Read the model definition and answer for the solid it produces. Units are mm, in the model's axes. Face numbers are marked on the shaded views. A direction names the side the tool comes from. Coordinates: 2 decimals unless noted, no trailing zeros. Write each loop counter-clockwise with the first axis right and the second up, starting at its lowest first coordinate (ties: lowest second). Pieces come first, ordered by that corner, then holes. Notation, with made-up numbers: (23, -7.5) -> (39, -7.5) arc R27 ccw to (39, 30.5) -> close; hole circle Ø8 at (54.25, -21). An arc over 180 degrees is marked (long way). Answer in a Markdown table with one row per item. Add a question column.
Item 1: For a pull along Y with two mould halves and no side action, classify the marked faces 5, 6, 7 and 8 as +Y half, -Y half, draft (parallel to the pull), parting line (faces both ways), or undercut.
Item 2: Which of the six approach directions +Z, -Z, +X, -X, +Y, -Y give full straight-line access (tool end or side, diameter ignored) to the marked faces 1, 2, 3 and 4?
Item 3: Given pin 1 Ø1.5 at (y, z) = (-1.5, 4) entering from -X; pin 2 Ø3.5 at (y, z) = (15, 4) entering from -X; pin 3 Ø3 at (x, z) = (5.5, 4) entering from -Y, each flat-ended and moving along its own axis, determine where each tip first touches the part or whether it passes through.
Item 4: Section A-A on x = 4.8 is taken. Write down the section's boundary in (y, z).
Item 5: Section D-D on z = 3.5 is taken. Count the separate pieces of the cut face and the enclosed holes in it, then the cut area to 3 significant figures.
Item 6: Section C-C on y = 0 is taken. Write down the section's boundary in (x, z).
Item 7: Section B-B on y = 18.5 is taken. Write down the section's boundary in (x, z).
Item 8: Straight lines are drawn through the part: line 1 (Z direction, x = 4.8, y = 13.25); line 2 (Y direction, x = -0.25, z = 2.25); line 3 (Y direction, x = 8, z = 0.75). For each, find the intervals that lie inside material, in ascending order. Write a range as from..to.
```python
from build123d import *

# Parameters (mm, degrees)
BOSS_EXTRUDE1_DEPTH = 8
SKETCH2_R           = 1.65
CUT_EXTRUDE1_DEPTH  = 18
CUT_EXTRUDE2_DEPTH  = 2.3
SKETCH5_W           = 8.4
SKETCH5_H           = 8
SKETCH5_R           = 1.65
BOSS_EXTRUDE2_DEPTH = 16.1
FILLET1_R           = 10
FILLET2_R           = 2
CHAMFER1_SIZE       = 0.5


with BuildPart() as part:
    # Sketch1 → Boss-Extrude1 (new body)
    with BuildSketch(Plane.XY):
        with BuildLine():
            Line((0, 6), (9, 6))
            Line((9, 6), (9, 2.552710574))
            Line((9, 2.552710574), (1.929680991, 2.552710574))
            ThreePointArc((1.929680991, 2.552710574), (-3.2, 0), (1.929680991, -2.552710574))
            Line((1.929680991, -2.552710574), (9, -2.552710574))
            Line((9, -2.552710574), (9, -6))
            Line((9, -6), (0, -6))
            ThreePointArc((0, -6), (-6, 0), (0, 6))
        make_face()
    extrude(amount=BOSS_EXTRUDE1_DEPTH)

    # Sketch2 → Cut-Extrude1 (cut, through all)
    with BuildSketch(Plane.XZ.offset(6)):
        with Locations(Location((4.8, 4, 0), (0, 0, 270))):
            Circle(SKETCH2_R)
    extrude(amount=-CUT_EXTRUDE1_DEPTH, mode=Mode.SUBTRACT)

    # Sketch3 → Cut-Extrude2 (cut)
    with BuildSketch(Plane.XZ.offset(6)):
        Polygon((6.4, 6.771281292), (3.2, 6.771281292), (1.6, 4), (3.2, 1.228718708), (6.4, 1.228718708), (8, 4), align=None)
    extrude(amount=-CUT_EXTRUDE2_DEPTH, mode=Mode.SUBTRACT)

    # Sketch5 → Boss-Extrude2 (add)
    with BuildSketch(Plane(origin=(0, 6, 0), x_dir=(1, 0, 0), z_dir=(0, 1, 0))):
        with Locations((4.8, -4)):
            Rectangle(SKETCH5_W, SKETCH5_H)
        with Locations(Location((4.8, -4, 0), (0, 0, 90))):
            Circle(SKETCH5_R, mode=Mode.SUBTRACT)
    extrude(amount=BOSS_EXTRUDE2_DEPTH)

    # Fillet1
    fillet1_edges = [part.edges().sort_by_distance(p)[0] for p in [
        (0.6, 6, 4),
    ]]
    fillet(fillet1_edges, radius=FILLET1_R)

    # Fillet2
    fillet2_edges = [part.edges().sort_by_distance(p)[0] for p in [
        (9, 22.1, 4),
        (0.6, 22.1, 4),
    ]]
    fillet(fillet2_edges, radius=FILLET2_R)

    # Chamfer1
    chamfer1_edges = [part.edges().sort_by_distance(p)[0] for p in [
        (5.464840496, 2.552710574, 0),
        (-3.2, 0, 0),
        (-5.706665837, -1.853096064, 0),
        (-0.490735159, 8.406111117, 0),
        (4.8, 22.1, 0),
        (5.464840496, -2.552710574, 0),
        (0.6, 16.523793324, 0),
        (1.185786438, 21.514213562, 0),
        (8.414213562, 21.514213562, 0),
        (9, -4.276355287, 0),
        (4.5, -6, 0),
        (9, 11.326355287, 0),
    ]]
    chamfer(chamfer1_edges, length=CHAMFER1_SIZE)


solid = part.part
```
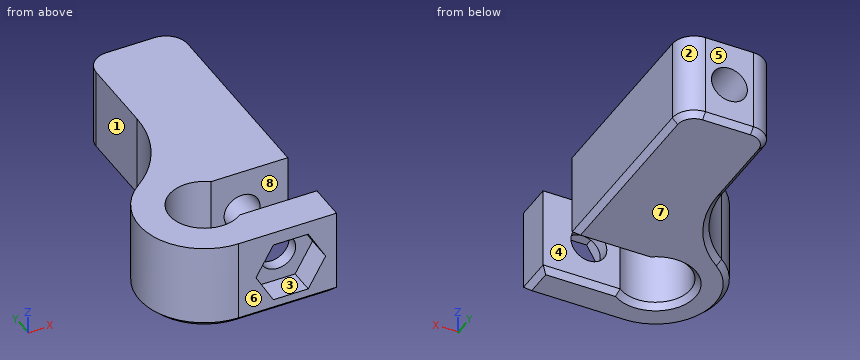
Results below:
| question | item | result |
|---|---|---|
| 1 | face 5 | +Y half |
| 1 | face 6 | -Y half |
| 1 | face 7 | draft |
| 1 | face 8 | undercut |
| 2 | face 1 | +Z, -Z, -X, +Y |
| 2 | face 2 | +Z, -Z, +X, +Y |
| 2 | face 3 | -Y |
| 2 | face 4 | +Z, -Z, +X |
| 3 | pin 1 | stops at x = -5.95 |
| 3 | pin 2 | stops at x = 0.6 |
| 3 | pin 3 | stops at y = -3.7 |
| 4 | outline | (-6, 0.5) -> (-5.5, 0) -> (-3.05, 0) -> (-2.55, 0.5) -> (-2.55, 2.35) -> (-3.7, 2.35) -> (-3.7, 1.23) -> (-6, 1.23) -> close; (-6, 6.77) -> (-3.7, 6.77) -> (-3.7, 5.65) -> (-2.55, 5.65) -> (-2.55, 8) -> (-6, 8) -> close; (2.55, 0.5) -> (3.05, 0) -> (21.6, 0) -> (22.1, 0.5) -> (22.1, 2.35) -> (2.55, 2.35) -> close; (2.55, 5.65) -> (22.1, 5.65) -> (22.1, 8) -> (2.55, 8) -> close |
| 5 | separate pieces | 3 |
| 5 | enclosed holes | 0 |
| 5 | area | 162 mm2 |
| 6 | outline | (-6, 0.5) -> (-5.5, 0) -> (-3.7, 0) -> (-3.2, 0.5) -> (-3.2, 8) -> (-6, 8) -> close |
| 7 | outline | (0.6, 0.5) -> (1.1, 0) -> (8.5, 0) -> (9, 0.5) -> (9, 8) -> (0.6, 8) -> close; hole circle Ø3.3 at (4.8, 4) |
| 8 | line 1 | z = 0..2.35, 5.65..8 |
| 8 | line 2 | y = -5.99..-3.19, 3.19..8.91 |
| 8 | line 3 | y = -6..-2.55, 2.55..21.83 |
